from build123d import *

# Parameters (mm, degrees)
BOSS_EXTRU_1_DEPTH = 6


with BuildPart() as part:
    # Esquisse1 → Boss.-Extru.1 (new body)
    with BuildSketch(Plane.XY):
        Polygon((-17.337221854, 10.148336377), (-17.337221854, 7.748336377), (-18.950778827, 6.252865249), (-17.337221854, 4.757394121), (-17.337221854, 2.357394121), (-14.937221854, 2.357394121), (-13.441750726, 0.743837148), (-11.946279598, 2.357394121), (-9.546279598, 2.357394121), (-9.546279598, 4.757394121), (-7.932722625, 6.252865249), (-9.546279598, 7.748336377), (-9.546279598, 10.148336377), (-11.946279598, 10.148336377), (-13.441750726, 11.761893351), (-14.937221854, 10.148336377), align=None)
        with BuildLine():
            Line((-16.039826937, 4.752865249), (-16.039826937, 7.752865249))
            ThreePointArc((-16.039826937, 7.752865249), (-10.441750726, 6.252865249), (-16.039826937, 4.752865249))
        make_face(mode=Mode.SUBTRACT)
    extrude(amount=BOSS_EXTRU_1_DEPTH)


solid = part.part
The listing builds one solid part. Answer for the finished solid, in the listing's coordinates (mm). A direction names the side the tool comes from. Give positions to 0.01 mm unless a question says otherwise; leave off trailing zeros. Write each loop counter-clockwise with the first axis right and the second up, starting at its lowest first coordinate (ties: lowest second). Pieces come first, ordered by that corner, then holes. Notation, with made-up numbers: (-20.75, 16.5) - (-13.75, 16.5) arc R14 cw to (-13.75, 40.5) - close; hole circle Ø9 at (82.25, -14.5). An arc over 180 degrees is marked (long way). One line per question, with ' | ' between items. Start each with the question number.
1. Section A-A, the plane z = 2.5 is taken. Determine the outline of the cut face in (x, y).
2. Section D-D, the plane x = -8.5 is taken. Determine the outline of the cut face in (y, z).
3. Straight lines are drawn through the part: line 1 (Y direction, x = -14, z = 3.8); line 2 (Y direction, x = -14.5, z = 0.45); line 3 (X direction, y = 3.5, z = 0.65). For each, find the intervals that lie inside material, in ascending order.
4. For faces 1 (the face through (-9.546, 9, 3)), 2 (the face through (-11, 2.357, 3)), 3 (the face through (-18.16, 5.52, 2.96)), 4 (the face through (-16, 10.148, 3)), determine the directions among +Z, -Z, +X, -X, +Y, -Y from which every point of the face is accessible in a straight line to the end or side of a thin tool.
5. Section C-C, the plane y = 3.75 is taken. Determine the outline of the cut face in (x, z).
6. Given P1, Ø0.7, axis at x = -16, z = 2, coming from the -Y side; P2, Ø3, axis at x = -16, z = 4.5, coming from the +Y side; P3, Ø0.7, axis at y = 3.5, z = 2, coming from the -X side, each flat-ended and moving along its own axis, determine where each tip first touches the part or whether it passes through.
7. Section B-B, the plane x = -11 is taken. Determine the outline of the cut face in (y, z).
8. Determine the mould class of faces 5 (the face through (-16, 2.357, 3)), 6 (the face through (-17.337, 4, 3)), 7 (the face through (-10.444, 6.363, 2.958)) for opening direction X: +X half, -X half, draft (parallel to the pull), parting line (faces both ways), or undercut.
Result:
1) outline: (-18.95, 6.25) - (-17.34, 4.76) - (-17.34, 2.36) - (-14.94, 2.36) - (-13.44, 0.74) - (-11.95, 2.36) - (-9.55, 2.36) - (-9.55, 4.76) - (-7.93, 6.25) - (-9.55, 7.75) - (-9.55, 10.15) - (-11.95, 10.15) - (-13.44, 11.76) - (-14.94, 10.15) - (-17.34, 10.15) - (-17.34, 7.75) - close; hole (-16.04, 4.75) arc R3 ccw (long way) to (-16.04, 7.75) - close
2) outline: (5.73, 0) - (6.78, 0) - (6.78, 6) - (5.73, 6) - close
3) line 1: y = 1.35 to 3.31, 9.2 to 11.16 | line 2: y = 1.89 to 3.45, 9.06 to 10.62 | line 3: x = -17.34 to -14.63, -12.25 to -9.55
4) face 1: +Z, -Z, +X, +Y | face 2: +Z, -Z, +X, -Y | face 3: +Z, -Z, -X, -Y | face 4: +Z, -Z, -X, +Y
5) outline: (-17.34, 0) - (-15.1, 0) - (-15.1, 6) - (-17.34, 6) - close; (-11.79, 0) - (-9.55, 0) - (-9.55, 6) - (-11.79, 6) - close
6) P1: stops at y = 2.36 | P2: stops at y = 10.62 | P3: stops at x = -17.34
7) outline: (2.36, 0) - (4.51, 0) - (4.51, 6) - (2.36, 6) - close; (8, 0) - (10.15, 0) - (10.15, 6) - (8, 6) - close
8) face 5: draft | face 6: -X half | face 7: undercut
